Check sheet for the modelled part. Datum: model origin and axes. Units: mm. A direction names the side the tool comes from. Give positions to 0.01 mm unless a question says otherwise; leave off trailing zeros. Answer as a JSON object with one key per item and string values.
from build123d import *

# Parameters (mm, degrees)
SKETCH2_W           = 570
SKETCH2_H           = 390
BOSS_EXTRUDE1_DEPTH = 22
SKETCH4_W           = 534
SKETCH4_H           = 10
CUT_EXTRUDE1_DEPTH  = 378
SKETCH5_W           = 12
SKETCH5_H           = 10
BOSS_EXTRUDE2_DEPTH = 378
CUT_EXTRUDE3_REACH  = 572
SKETCH6_R           = 2.5
CUT_EXTRUDE4_REACH  = 572
SKETCH7_R           = 2.5
SKETCH3_W           = 52
SKETCH3_H           = 362
CUT_EXTRUDE5_DEPTH  = 23


with BuildPart() as part:
    # Sketch2 → Boss-Extrude1 (new body)
    with BuildSketch(Plane.XY):
        Rectangle(SKETCH2_W, SKETCH2_H)
    extrude(amount=BOSS_EXTRUDE1_DEPTH)

    # Sketch4 → Cut-Extrude1 (cut)
    with BuildSketch(Plane(origin=(0, 195, 0), x_dir=(1, 0, 0), z_dir=(0, 1, 0))):
        with Locations((0, -11)):
            Rectangle(SKETCH4_W, SKETCH4_H)
    extrude(amount=-CUT_EXTRUDE1_DEPTH, mode=Mode.SUBTRACT)

    # Sketch5 → Boss-Extrude2 (add)
    with BuildSketch(Plane(origin=(0, 195, 0), x_dir=(1, 0, 0), z_dir=(0, 1, 0))):
        with Locations((195, -11)):
            Rectangle(SKETCH5_W, SKETCH5_H)
        with Locations((117, -11)):
            Rectangle(SKETCH5_W, SKETCH5_H)
        with Locations((39, -11)):
            Rectangle(SKETCH5_W, SKETCH5_H)
        with Locations((-39, -11)):
            Rectangle(SKETCH5_W, SKETCH5_H)
        with Locations((-117, -11)):
            Rectangle(SKETCH5_W, SKETCH5_H)
        with Locations((-195, -11)):
            Rectangle(SKETCH5_W, SKETCH5_H)
    extrude(amount=-BOSS_EXTRUDE2_DEPTH)

    # Sketch6 → Cut-Extrude3 (cut, up to next)
    with BuildSketch(Plane.ZY.offset(285), mode=Mode.PRIVATE) as cut_extrude3_sk1:
        with Locations((11, 1)):
            Circle(SKETCH6_R)
    cut_extrude3_tool1 = extrude(cut_extrude3_sk1.sketch, amount=-CUT_EXTRUDE3_REACH, mode=Mode.PRIVATE) & part.part
    add(cut_extrude3_tool1.solids().sort_by_distance((-285, 1, 11))[0], mode=Mode.SUBTRACT)

    # Sketch7 → Cut-Extrude4 (cut, up to next)
    with BuildSketch(Plane(origin=(285, 0, 0), x_dir=(0, 0, -1), z_dir=(1, 0, 0)), mode=Mode.PRIVATE) as cut_extrude4_sk1:
        with Locations((-11, 1)):
            Circle(SKETCH7_R)
    cut_extrude4_tool1 = extrude(cut_extrude4_sk1.sketch, amount=-CUT_EXTRUDE4_REACH, mode=Mode.PRIVATE) & part.part
    add(cut_extrude4_tool1.solids().sort_by_distance((285, 1, 11))[0], mode=Mode.SUBTRACT)

    # Sketch3 → Cut-Extrude5 (cut, through all)
    with BuildSketch(Plane(origin=(0, 0, 0), x_dir=(-1, 0, 0), z_dir=(0, 0, -1))):
        with Locations((-156, 2)):
            Rectangle(SKETCH3_W, SKETCH3_H)
        with Locations((-234, 2)):
            Rectangle(SKETCH3_W, SKETCH3_H)
        with Locations((-78, 2)):
            Rectangle(SKETCH3_W, SKETCH3_H)
        with Locations((0, 2)):
            Rectangle(SKETCH3_W, SKETCH3_H)
        with Locations((78, 2)):
            Rectangle(SKETCH3_W, SKETCH3_H)
        with Locations((156, 2)):
            Rectangle(SKETCH3_W, SKETCH3_H)
        with Locations((234, 2)):
            Rectangle(SKETCH3_W, SKETCH3_H)
    extrude(amount=-CUT_EXTRUDE5_DEPTH, mode=Mode.SUBTRACT)


solid = part.part
1. Access from +Z, -Z, +X, -X, +Y, -Y to the whole of each face (thin tool, end or side, straight path). Record for faces 5 (the face through (-4, -195, 11)), 6 (the face through (51, 35, 6)).
Determined:
{"face 5": "+Z, -Z, +X, -X, -Y", "face 6": "+Y"}
2. Go/stop test with a flat-tipped pin: P1, Ø20, axis at x = -68, y = -48, coming from the -Z side. Record where the tip stops, or that it passes through.
Determined:
{"P1": "through"}
3. Sectioned sample at A-A, the plane y = -19. State how many separate pieces and enclosed holes the cut face has, plus the area to 3 significant figures.
Determined:
{"separate pieces": "8", "enclosed holes": "0", "area": "3,550 mm^2"}
4. Mould release check, pull along X, two halves, no side actions. Record for faces 1 (the face through (-285, -3, 11)), 2 (the face through (-261, 35, 16)), 3 (the face through (-44, 15, 22)), 4 (the face through (-105, 35, 6)): released by +X, released by -X, zero draft, split by the parting line, or undercut.
Determined:
{"face 1": "released by -X", "face 2": "undercut", "face 3": "zero draft", "face 4": "undercut"}
5. Scan lines: L1, parallel to Y at x = -274, z = 11; L2, parallel to Z at x = -128, y = -17; L3, parallel to Y at x = -161, z = 9.5. Record each from-to range of solid material in increasing order. Write a range as [from, to].
Determined:
{"L1": "[-195, -1.5], [3.5, 195]", "L2": "[0, 6], [16, 22]", "L3": "[-195, -183]"}
